```python
from build123d import *

# Parameters (mm, degrees)
F0_R     = 2.25
F0_R_2   = 38.25
F1_DEPTH = 25.25
F2_R     = 16.5
F3_DEPTH = 25.25


with BuildPart() as f1:
    # F0 (on Top) → F1 (new body)
    with BuildSketch(Plane.XY):
        with BuildLine():
            Line((-37, -40), (37, -40))
            ThreePointArc((37, -40), (39.12132, -39.12132), (40, -37))
            Line((40, -37), (40, 37))
            ThreePointArc((40, 37), (39.12132, 39.12132), (37, 40))
            Line((37, 40), (-37, 40))
            ThreePointArc((-37, 40), (-39.12132, 39.12132), (-40, 37))
            Line((-40, 37), (-40, -37))
            ThreePointArc((-40, -37), (-39.12132, -39.12132), (-37, -40))
        make_face()
        with Locations((-35.75, -35.75)):
            Circle(F0_R, mode=Mode.SUBTRACT)
        with Locations((35.75, -35.75)):
            Circle(F0_R, mode=Mode.SUBTRACT)
        with Locations((-35.75, 35.75)):
            Circle(F0_R, mode=Mode.SUBTRACT)
        Circle(F0_R_2, mode=Mode.SUBTRACT)
        with Locations((35.75, 35.75)):
            Circle(F0_R, mode=Mode.SUBTRACT)
    extrude(amount=F1_DEPTH)


with BuildPart() as f3:
    # F2 (on Top) → F3 (new body)
    with BuildSketch(Plane.XY):
        Circle(F2_R)
    extrude(amount=F3_DEPTH)


solid = f1.part
```
CAD build for the part. Positions are in the model's coordinates, mm. Round coordinates to 2 decimals unless told otherwise and drop trailing zeros. Order: outer loops, then holes, each group sorted by start corner. A loop starts at its lowest first (then second) coordinate and runs counter-clockwise, first axis right, second up. Notation, with made-up numbers: (26.25, -14.5) - (66.25, -14.5) arc R17 cw to (66.25, 5.5) - close; hole circle Ø2 at (29.25, 11). An arc over 180 degrees is marked (long way). Answer as CSV lines item,"result". Start each with the question number.
1. Pull direction Y, two halves, no side cores. Call faces 1 (the face through (-20.9, -32.4, 0)), 2 (the face through (-39.14, -39.1, 12.45)), 3 (the face through (-34.54, -33.853, 12.448)), 4 (the face through (1, 40, 12)): +Y half, -Y half, draft (parallel to the pull), parting line (faces both ways), or undercut.
2. Saw through at A-A, the plane x = 0. Write the cut outline in (y, z), and give its area (3 significant figures).
3. Saw through at D-D, the plane y = 35.75. Write the cut outline in (x, z).
4. Drill centre lines: L1, parallel to Y at x = 0, z = 9.25; L2, parallel to X at y = 30, z = 23.75. Where is each one in solid material? Low to high. Write a range as [from, to].
5. Saw through at C-C, the plane z = 16. Write the cut outline in (x, y).
Model answer:
1,face 1,"draft"
1,face 2,"-Y half"
1,face 3,"undercut"
1,face 4,"+Y half"
2,outline,"(-40, 0) - (-38.25, 0) - (-38.25, 25.25) - (-40, 25.25) - close; (38.25, 0) - (40, 0) - (40, 25.25) - (38.25, 25.25) - close"
2,area,"88.4 mm²"
3,outline,"(-40, 0) - (-38, 0) - (-38, 25.25) - (-40, 25.25) - close; (-33.5, 0) - (-13.6, 0) - (-13.6, 25.25) - (-33.5, 25.25) - close; (13.6, 0) - (33.5, 0) - (33.5, 25.25) - (13.6, 25.25) - close; (38, 0) - (40, 0) - (40, 25.25) - (38, 25.25) - close"
4,L1,"y = [-40, -38.25], [38.25, 40]"
4,L2,"x = [-40, -23.73], [23.73, 40]"
5,outline,"(-40, -37) arc R3 ccw to (-37, -40) - (37, -40) arc R3 ccw to (40, -37) - (40, 37) arc R3 ccw to (37, 40) - (-37, 40) arc R3 ccw to (-40, 37) - close; hole circle Ø76.5 at (0, 0); hole circle Ø4.5 at (-35.75, -35.75); hole circle Ø4.5 at (-35.75, 35.75); hole circle Ø4.5 at (35.75, -35.75); hole circle Ø4.5 at (35.75, 35.75)"
